Geometry: see drawing. Coordinates: mm, zero at the bounding-box minimum. Coordinates: 2 decimals unless noted, no trailing zeros. Order: outer loops, then holes, each group sorted by start corner. A loop starts at its lowest first (then second) coordinate and runs counter-clockwise, first axis right, second up.
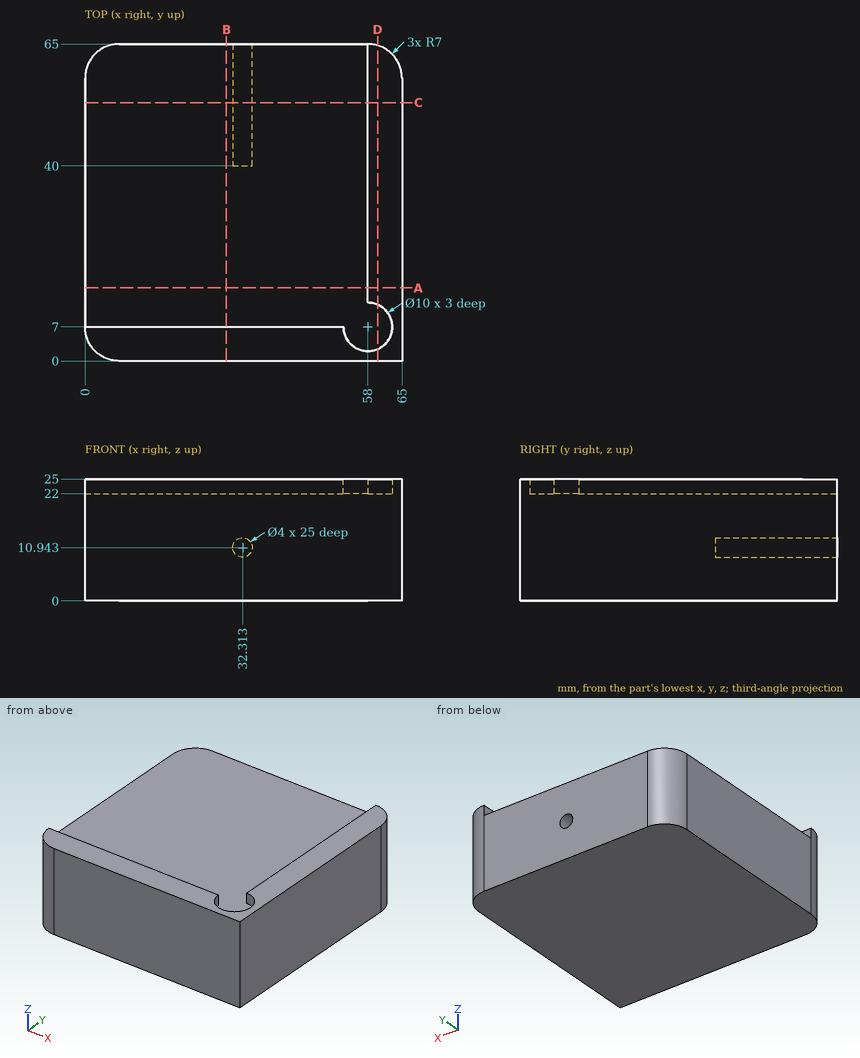
Item 1: Cut plane D-D on x = 60. Return loops of the section in (y, z).
Response values:
outline: (0, 0) - (64.71, 0) - (64.71, 25) - (11.58, 25) - (11.58, 22) - (2.42, 22) - (2.42, 25) - (0, 25) - close
Item 2: Cut plane A-A on y = 15. Return loops of the section in (x, z), then the cut area to 3 significant figures.
Response values:
outline: (0, 0) - (65, 0) - (65, 25) - (58, 25) - (58, 22) - (0, 22) - close
area: 1,450 mm2
Item 3: Pin query (flat end, axial travel): pin 1 Ø10 at (y, z) = (14.5, 11) entering from -X; pin 2 Ø12 at (x, y) = (16.5, 22) entering from +Z; pin 3 Ø1.5 at (x, z) = (33.5, 23.5) entering from +Y; pin 4 Ø0.9 at (y, z) = (33, 23.5) entering from -X. Return the tip coordinate at first contact, or that it passes through.
Response values:
pin 1: stops at x = 0
pin 2: stops at z = 22
pin 3: stops at y = 7
pin 4: stops at x = 58
Item 4: Ray query, probe 1 along Z at (x, y) = (51, 47); probe 2 along X at (y, z) = (56.5, 23.25); probe 3 along Y at (x, z) = (17, 23.5). Return the intervals inside material, ascending.
Response values:
probe 1: z = 0 to 22
probe 2: x = 58 to 65
probe 3: y = 0 to 7
Item 5: Cut plane B-B on x = 29. Return loops of the section in (y, z).
Response values:
outline: (0, 0) - (65, 0) - (65, 22) - (7, 22) - (7, 25) - (0, 25) - close
Item 6: Cut plane C-C on y = 53. Return loops of the section in (x, z), then the cut area to 3 significant figures.
Response values:
outline: (0, 0) - (65, 0) - (65, 25) - (58, 25) - (58, 22) - (0, 22) - close; hole circle Ø4 at (32.31, 10.94)
area: 1,440 mm2
